```python
from build123d import *

# Parameters (mm, degrees)
SKETCH1_W           = 137.16
SKETCH1_H           = 152.4
BOSS_EXTRUDE2_DEPTH = 25.4
CUT_EXTRUDE1_DEPTH  = 25.4
SKETCH2_R           = 2.2479
CUT_EXTRUDE2_DEPTH  = 25.4
FILLET2_R           = 25.4
FILLET3_R           = 19.05
FILLET4_R           = 127
CUT_EXTRUDE3_DEPTH  = 20.955
CHAMFER1_SIZE       = 1.016


with BuildPart() as part:
    # Sketch1 → Boss-Extrude2 (new body)
    with BuildSketch(Plane(origin=(0, 0, 0), x_dir=(1, 0, 0), z_dir=(0, 1, 0))):
        Rectangle(SKETCH1_W, SKETCH1_H)
    extrude(amount=-BOSS_EXTRUDE2_DEPTH)

    # Sketch3 → Cut-Extrude1 (cut)
    with BuildSketch(Plane(origin=(0, 0, 0), x_dir=(1, 0, 0), z_dir=(0, 1, 0))):
        with BuildLine():
            Line((68.58, 0), (59.262686671, -33.820874717))
            ThreePointArc((59.262686671, -33.820874717), (59.713399713, -40.366937171), (64.156526503, -45.195259885))
            ThreePointArc((64.156526503, -45.195259885), (67.293603318, -52.486532428), (60.865154116, -57.142598053))
            ThreePointArc((60.865154116, -57.142598053), (54.576224637, -59.014346409), (50.836773359, -64.406060426))
            Line((50.836773359, -64.406060426), (47.587660753, -76.2))
            Line((47.587660753, -76.2), (68.58, -76.2))
            Line((68.58, -76.2), (68.58, 0))
        make_face()
        with BuildLine():
            Line((-54.821666667, -47.612294916), (-54.821666667, -76.2))
            Line((-54.821666667, -76.2), (-68.58, -76.2))
            Line((-68.58, -76.2), (-68.58, 0))
            Line((-68.58, 0), (-54.821666667, 0))
            Line((-54.821666667, 0), (-54.821666667, -15.887705084))
            ThreePointArc((-54.821666667, -15.887705084), (-56.994797895, -22.078955084), (-62.560729167, -25.553791048))
            ThreePointArc((-62.560729167, -25.553791048), (-67.521666667, -31.75), (-62.560729167, -37.946208952))
            ThreePointArc((-62.560729167, -37.946208952), (-56.994797895, -41.421044916), (-54.821666667, -47.612294916))
        make_face()
    cut_extrude1 = extrude(amount=-CUT_EXTRUDE1_DEPTH, mode=Mode.SUBTRACT)

    # Mirror1: Cut-Extrude1 across plane
    add(cut_extrude1.mirror(Plane(origin=(-54.821666667, -104.438713977, 0), x_dir=(1, 0, 0), z_dir=(0, 0, -1))), mode=Mode.SUBTRACT)

    # Sketch2 → Cut-Extrude2 (cut)
    with BuildSketch(Plane(origin=(0, 0, 0), x_dir=(1, 0, 0), z_dir=(0, 1, 0))):
        with Locations(Location((-61.171666667, 31.75, 0), (0, 0, 270))):
            Circle(SKETCH2_R)
        with Locations(Location((-61.171666667, -31.75, 0), (0, 0, 270))):
            Circle(SKETCH2_R)
        with Locations(Location((61.171666667, 50.8, 0), (0, 0, 270))):
            Circle(SKETCH2_R)
        with Locations(Location((61.171666667, -50.8, 0), (0, 0, 270))):
            Circle(SKETCH2_R)
    extrude(amount=-CUT_EXTRUDE2_DEPTH, mode=Mode.SUBTRACT)

    # Fillet2
    fillet2_edges = [part.edges().sort_by_distance(p)[0] for p in [
        (-54.821666667, -12.7, 76.2),
        (-54.821666667, -12.7, -76.2),
    ]]
    fillet(fillet2_edges, radius=FILLET2_R)

    # Fillet3
    fillet3_edges = [part.edges().sort_by_distance(p)[0] for p in [
        (47.587660753, -12.7, 76.2),
        (47.587660753, -12.7, -76.2),
    ]]
    fillet(fillet3_edges, radius=FILLET3_R)

    # Fillet4
    fillet4_edges = [part.edges().sort_by_distance(p)[0] for p in [
        (68.58, -12.7, 0),
    ]]
    fillet(fillet4_edges, radius=FILLET4_R)

    # Sketch4 → Cut-Extrude3 (cut)
    with BuildSketch(Plane(origin=(0, 0, 0), x_dir=(1, 0, 0), z_dir=(0, 1, 0))):
        with BuildLine():
            Line((-50.376666667, 50.8), (-50.376666667, -50.8))
            ThreePointArc((-50.376666667, -50.8), (-44.239089266, -65.6174226), (-29.421666667, -71.755))
            Line((-29.421666667, -71.755), (29.421666667, -71.755))
            ThreePointArc((29.421666667, -71.755), (44.239089266, -65.6174226), (50.376666667, -50.8))
            Line((50.376666667, -50.8), (50.376666667, 50.8))
            ThreePointArc((50.376666667, 50.8), (44.239089266, 65.6174226), (29.421666667, 71.755))
            Line((29.421666667, 71.755), (-29.421666667, 71.755))
            ThreePointArc((-29.421666667, 71.755), (-44.239089266, 65.6174226), (-50.376666667, 50.8))
        make_face()
    extrude(amount=-CUT_EXTRUDE3_DEPTH, mode=Mode.SUBTRACT)

    # Chamfer1
    chamfer1_edges = [part.edges().sort_by_distance(p)[0] for p in [
        (44.239089266, 0, 65.6174226),
        (50.376666667, 0, 0),
        (44.239089266, 0, -65.6174226),
        (0, 0, -71.755),
        (-44.239089266, 0, -65.6174226),
        (-50.376666667, 0, 0),
        (-44.239089266, 0, 65.6174226),
        (0, 0, 71.755),
    ]]
    chamfer(chamfer1_edges, length=CHAMFER1_SIZE)


solid = part.part
```
The model under review builds one solid part; all positions refer to its coordinate system, in mm. A direction names the side the tool comes from. Coordinates: 2 decimals unless noted, no trailing zeros. Write each loop counter-clockwise with the first axis right and the second up, starting at its lowest first coordinate (ties: lowest second). Pieces come first, ordered by that corner, then holes. Notation, with made-up numbers: (-1.75, -33) -> (10.25, -33) arc R36 cw to (10.25, 3) -> close; hole circle Ø4 at (-36, -22.75). An arc over 180 degrees is marked (long way). One line per item, written item: value. Start each with the question number.
Q1. Add section C-C, the plane z = -21. Give the boundary of the cut face in (x, y) (3 decimals), then the cut area to 3 significant figures.
Q2. For faces 4 (the face through (-54.822, -13, -49)), 5 (the face through (44.401, -10.846, -65.454)), 6 (the face through (-54.822, -13, 0)), list the 3-axis set-ups (+Z, -Z, +X, -X, +Y, -Y) from which the entire face can be reached by the end or side of a thin tool; tool diameter is ignored.
Q3. Add section A-A, the plane z = 31.75. Give the boundary of the cut face in (x, y) (3 decimals).
Q4. The part is to be moulded in two halves that separate along Z. For faces 1 (the face through (-47.58, -12.88, -68.56)), 2 (the face through (-44.19, -0.85, -65.9)), 3 (the face through (-1, -25.4, -1)), say which applies: +Z half, -Z half, draft (parallel to the pull), parting line (faces both ways), or undercut.
Q5. Add section B-B, the plane x = 0.5. Give the boundary of the cut face in (y, z) (3 decimals), then the cut area to 3 significant figures.
Q6. To check wall thickness, follow probe 1 along X at (y, z) = (-9, 51); probe 2 along X at (y, z) = (-7.25, -31.75); probe 3 along Z at (x, y) = (-14.5, -16.75) (3 decimals). State the ranges of each line that lie inside material, in increasing order.
Q7. Clearance check with flat-ended pins moving along their axes: P1, Ø2, axis at y = -21.5, z = 34, coming from the +X side; P2, Ø8, axis at y = -7.5, z = 13.5, coming from the +X side; P3, Ø4, axis at y = -12.5, z = 23, coming from the +X side. State where each tip first meets the part, or that it passes through.
Q8. Add section D-D, the plane y = -18.75. Count the separate pieces of the cut face and the enclosed holes in it, then the cut area to 3 significant figures.
Response:
1. outline: (-56.243, -25.4) -> (62.101, -25.4) -> (62.101, 0) -> (51.393, 0) -> (50.377, -1.016) -> (50.377, -20.955) -> (-50.377, -20.955) -> (-50.377, -1.016) -> (-51.393, 0) -> (-56.243, 0) -> close
1. area: 894 mm²
2. face 4: -Z, -X, +Y, -Y
2. face 5: +Y
2. face 6: -X, +Y, -Y
3. outline: (-67.522, -25.4) -> (-63.42, -25.4) -> (-63.42, 0) -> (-67.522, 0) -> close; (-58.924, -25.4) -> (59.816, -25.4) -> (59.816, 0) -> (51.393, 0) -> (50.377, -1.016) -> (50.377, -20.955) -> (-50.377, -20.955) -> (-50.377, -1.016) -> (-51.393, 0) -> (-58.924, 0) -> close
4. face 1: -Z half
4. face 2: undercut
4. face 3: draft
5. outline: (-25.4, -76.2) -> (0, -76.2) -> (0, -72.771) -> (-1.016, -71.755) -> (-20.955, -71.755) -> (-20.955, 71.755) -> (-1.016, 71.755) -> (0, 72.771) -> (0, 76.2) -> (-25.4, 76.2) -> close
5. area: 863 mm²
6. probe 1: -54.82 to -50.38, 50.38 to 58.93, 63.41 to 67.52
6. probe 2: -67.52 to -63.42, -58.92 to -50.38, 50.38 to 59.82
6. probe 3: -76.2 to -71.755, 71.755 to 76.2
7. P1: x = 59.49
7. P2: x = 63.49
7. P3: x = 62.1
8. separate pieces: 1
8. enclosed holes: 5
8. area: 3,320 mm²
